Source: CAD feature listing. Evaluate the final solid. Frame: model axes, mm. Face numbers are marked on the shaded views. A direction names the side the tool comes from. Give positions to 0.01 mm unless a question says otherwise; leave off trailing zeros. Write each loop counter-clockwise with the first axis right and the second up, starting at its lowest first coordinate (ties: lowest second). Pieces come first, ordered by that corner, then holes. Notation, with made-up numbers: (4.25, -27.75) - (45.25, -27.75) arc R20 ccw to (45.25, -12.75) - close; hole circle Ø3 at (72, 26.25). An arc over 180 degrees is marked (long way). Answer as a JSON object with one key per item and string values. Group by question number.
from build123d import *

# Parameters (mm, degrees)
BOSS_EXTRUDE1_DEPTH      = 120
BOSS_EXTRUDE1_DEPTH_BACK = 30
SKETCH1_W                = 28
SKETCH1_H                = 28
CHAMFER1_SIZE            = 18
SKETCH2_W                = 150
SKETCH2_H                = 28
BOSS_EXTRUDE2_DEPTH      = 100
SKETCH3_W                = 142
SKETCH3_H                = 100
CUT_EXTRUDE1_DEPTH       = 24
SKETCH4_W                = 142
SKETCH4_H                = 20
CUT_EXTRUDE2_DEPTH       = 4
CHAMFER2_SIZE            = 20
SKETCH6_R                = 1.75
CUT_EXTRUDE3_DEPTH       = 171.064693573
SKETCH10_W               = 165.029573665
SKETCH10_H               = 25.818236019
CUT_EXTRUDE7_DEPTH       = 168.868996542
CUT_EXTRUDE8_DEPTH       = 180.931301028
CHAMFER3_SIZE            = 3
SKETCH12_W               = 142
SKETCH12_H               = 11.455844122
CUT_EXTRUDE9_DEPTH       = 160.52775952
SKETCH13_W               = 142
SKETCH13_H               = 6
BOSS_EXTRUDE4_DEPTH      = 24
SKETCH14_R               = 2.25
CUT_EXTRUDE10_DEPTH      = 6
SKETCH15_R               = 1.75
CUT_EXTRUDE11_DEPTH      = 177.610512398
SKETCH17_R               = 3.5
BOSS_EXTRUDE5_DEPTH      = 3
SKETCH18_R               = 2.1
CUT_EXTRUDE12_DEPTH      = 6


with BuildPart() as part:
    # Sketch1 → Boss-Extrude1 (new, two sides: drawn at the far end of the back side and taken through both)
    with BuildSketch(Plane(origin=(0, 0, 0), x_dir=(0, 0, -1), z_dir=(1, 0, 0)).offset(-BOSS_EXTRUDE1_DEPTH_BACK)):
        Rectangle(SKETCH1_W, SKETCH1_H)
    extrude(amount=BOSS_EXTRUDE1_DEPTH + BOSS_EXTRUDE1_DEPTH_BACK)

    # Chamfer1
    chamfer1_edges = [part.edges().sort_by_distance(p)[0] for p in [
        (45, -14, 14),
    ]]
    chamfer(chamfer1_edges, length=CHAMFER1_SIZE)

    # Sketch2 → Boss-Extrude2 (add)
    with BuildSketch(Plane(origin=(0, 0, -14), x_dir=(-1, 0, 0), z_dir=(0, 0, -1))):
        with Locations((-45, 0)):
            Rectangle(SKETCH2_W, SKETCH2_H)
    extrude(amount=BOSS_EXTRUDE2_DEPTH)

    # Sketch3 → Cut-Extrude1 (cut)
    with BuildSketch(Plane(origin=(0, 14, 0), x_dir=(1, 0, 0), z_dir=(0, 1, 0))):
        with Locations((45, 60)):
            Rectangle(SKETCH3_W, SKETCH3_H)
    extrude(amount=-CUT_EXTRUDE1_DEPTH, mode=Mode.SUBTRACT)

    # Sketch4 → Cut-Extrude2 (cut)
    with BuildSketch(Plane(origin=(0, 14, 0), x_dir=(1, 0, 0), z_dir=(0, 1, 0))):
        with Locations((45, 0)):
            Rectangle(SKETCH4_W, SKETCH4_H)
    extrude(amount=-CUT_EXTRUDE2_DEPTH, mode=Mode.SUBTRACT)

    # Chamfer2
    chamfer2_edges = [part.edges().sort_by_distance(p)[0] for p in [
        (45, 10, -10),
    ]]
    chamfer(chamfer2_edges, length=CHAMFER2_SIZE - 0.0001)  # a hair under: the kernel refuses the full size

    # Sketch6 → Cut-Extrude3 (cut, through all)
    with BuildSketch(Plane(origin=(0, -5, 5), x_dir=(1, 0, 0), z_dir=(0, -0.7071067811865465, 0.7071067811865487))):
        with Locations(Location((34, 10, 0), (0, 0, 270))):
            Circle(SKETCH6_R)
        with Locations(Location((17.996557672, 10, 0), (0, 0, 270))):
            Circle(SKETCH6_R)
        with Locations(Location((56, 10, 0), (0, 0, 270))):
            Circle(SKETCH6_R)
        with Locations(Location((72, 10, 0), (0, 0, 270))):
            Circle(SKETCH6_R)
        with Locations(Location((72, -10, 0), (0, 0, 270))):
            Circle(SKETCH6_R)
        with Locations(Location((56, -10, 0), (0, 0, 270))):
            Circle(SKETCH6_R)
        with Locations(Location((34, -10, 0), (0, 0, 270))):
            Circle(SKETCH6_R)
        with Locations(Location((17.996557672, -10, 0), (0, 0, 270))):
            Circle(SKETCH6_R)
    extrude(amount=-CUT_EXTRUDE3_DEPTH, mode=Mode.SUBTRACT)

    # Sketch10 → Cut-Extrude7 (cut, through all)
    with BuildSketch(Plane(origin=(0, 14, 0), x_dir=(1, 0, 0), z_dir=(0, 1, 0))):
        with Locations((52.514786833, 111.292414811)):
            Rectangle(SKETCH10_W, SKETCH10_H)
    extrude(amount=-CUT_EXTRUDE7_DEPTH, mode=Mode.SUBTRACT)

    # Sketch11 → Cut-Extrude8 (cut, through all)
    with BuildSketch(Plane.ZY.offset(30)):
        Polygon((9.050252532, -0.949747468), (3.393398282, 4.707106781), (-4.707106781, -3.393398282), (0.949747468, -9.050252532), align=None)
    extrude(amount=-CUT_EXTRUDE8_DEPTH, mode=Mode.SUBTRACT)

    # Chamfer3
    chamfer3_edges = [part.edges().sort_by_distance(p)[0] for p in [
        (-28, 4.707106781, 3.393398282),
        (-28, -3.393398282, -4.707106781),
    ]]
    chamfer(chamfer3_edges, length=CHAMFER3_SIZE)

    # Sketch12 → Cut-Extrude9 (cut, through all)
    with BuildSketch(Plane(origin=(0, -5, 5), x_dir=(-1, 0, 0), z_dir=(0, -0.7071067811865513, 0.7071067811865437))):
        with Locations((-45, 0)):
            Rectangle(SKETCH12_W, SKETCH12_H)
    extrude(amount=-CUT_EXTRUDE9_DEPTH, mode=Mode.SUBTRACT)

    # Sketch13 → Boss-Extrude4 (add)
    with BuildSketch(Plane(origin=(0, -10, 0), x_dir=(1, 0, 0), z_dir=(0, 1, 0))):
        with Locations((45, 95.383296801)):
            Rectangle(SKETCH13_W, SKETCH13_H)
    extrude(amount=BOSS_EXTRUDE4_DEPTH)

    # Sketch14 → Cut-Extrude10 (cut)
    with BuildSketch(Plane(origin=(0, 0, -98.383296801), x_dir=(-1, 0, 0), z_dir=(0, 0, -1))):
        with Locations((-101, 2)):
            Circle(SKETCH14_R)
    extrude(amount=-CUT_EXTRUDE10_DEPTH, mode=Mode.SUBTRACT)

    # Sketch15 → Cut-Extrude11 (cut, through all)
    with BuildSketch(Plane(origin=(-26, 0, 0), x_dir=(0, 0, -1), z_dir=(1, 0, 0))):
        with Locations((88.383296801, 8)):
            Circle(SKETCH15_R)
        with Locations((88.383296801, -4)):
            Circle(SKETCH15_R)
    extrude(amount=-CUT_EXTRUDE11_DEPTH, mode=Mode.SUBTRACT)

    # Sketch17 → Boss-Extrude5 (add)
    with BuildSketch(Plane(origin=(0, -10, 0), x_dir=(1, 0, 0), z_dir=(0, 1, 0))):
        with Locations(Location((1, 84.383296801, 0), (0, 0, 270))):
            Circle(SKETCH17_R)
        with Locations(Location((84, 84.383296801, 0), (0, 0, 270))):
            Circle(SKETCH17_R)
        with Locations(Location((84, 27.383296801, 0), (0, 0, 270))):
            Circle(SKETCH17_R)
        with Locations(Location((1, 27.383296801, 0), (0, 0, 270))):
            Circle(SKETCH17_R)
    extrude(amount=BOSS_EXTRUDE5_DEPTH)

    # Sketch18 → Cut-Extrude12 (cut)
    with BuildSketch(Plane(origin=(0, -7, 0), x_dir=(1, 0, 0), z_dir=(0, 1, 0))):
        with Locations(Location((84, 84.383296801, 0), (0, 0, 270))):
            Circle(SKETCH18_R)
        with Locations(Location((84, 27.383296801, 0), (0, 0, 270))):
            Circle(SKETCH18_R)
        with Locations(Location((1, 27.383296801, 0), (0, 0, 270))):
            Circle(SKETCH18_R)
        with Locations(Location((1, 84.383296801, 0), (0, 0, 270))):
            Circle(SKETCH18_R)
    extrude(amount=-CUT_EXTRUDE12_DEPTH, mode=Mode.SUBTRACT)


solid = part.part
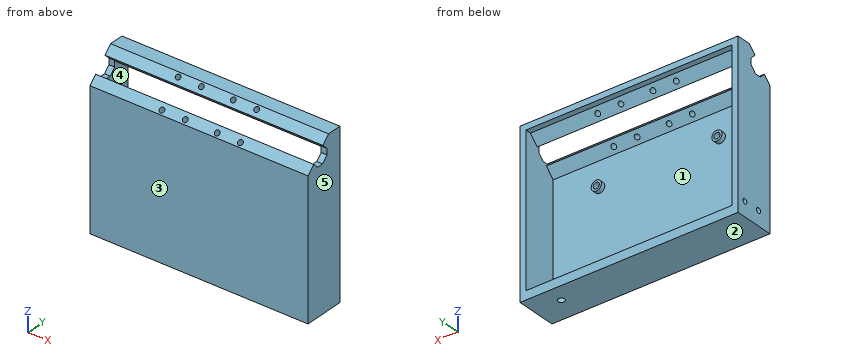
Q1. Reachability of the marked faces 1 and 2 from +Z, -Z, +X, -X, +Y, -Y: full face, straight path, thin tool, end or side. Return the list, or none.
Q2. First-contact query: pin 1 Ø2.5 at (x, z) = (84, -27.38) entering from +Y; pin 2 Ø3.5 at (x, y) = (101, 2) entering from -Z; pin 3 Ø10 at (x, z) = (94, -53) entering from +Y. Flat tips, straight axial feed; report the tip coordinate or a pass-through.
Q3. Draft query along X for the marked faces 3, 4 and 5. Return one class per face: released by +X, released by -X, zero draft, split by the parting line, or undercut.
Q4. Section B-B on y = 11.75. Return the cut outline in (x, z), then the cut area to 3 significant figures.
Q5. Section C-C on x = 101. State how many separate pieces and enclosed holes the cut face has, then the cut area to 3 significant figures.
Q6. Section D-D on z = -55.5. Return the cut outline in (x, y), then the cut area to 3 significant figures.
Q7. Ray query, probe 1 along X at (y, z) = (-6.5, -78.5); probe 2 along Z at (x, y) = (-15, 11.25); probe 3 along Z at (x, y) = (-14, -7). Return the intervals inside material, ascending. Write a range as [from, to].
Taken from the geometry:
{
 "1": {"face 1": "+Y", "face 2": "-Z, +X, -X, +Y, -Y"},
 "2": {"pin 1": "stops at y = -13", "pin 2": "stops at z = 4.35", "pin 3": "stops at y = -10"},
 "3": {"face 3": "zero draft", "face 4": "undercut", "face 5": "released by +X"},
 "4": {"outline": "(-30, -98.38) - (120, -98.38) - (120, 14) - (-30, 14) - close; hole (-26, -92.38) - (116, -92.38) - (116, 10) - (-26, 10) - close", "area": "2,320 mm²"},
 "5": {"separate pieces": "3", "enclosed holes": "0", "area": "620 mm²"},
 "6": {"outline": "(-30, -14) - (120, -14) - (120, 14) - (116, 14) - (116, -10) - (-26, -10) - (-26, 14) - (-30, 14) - close", "area": "792 mm²"},
 "7": {"probe 1": "x = [-30, -26], [116, 120]", "probe 2": "z = [-98.38, -92.38], [10, 14]", "probe 3": "z = [-98.38, -92.38], [-7, -1.1]"}
}
